Design review of the part built by this model. Coordinates are the model's own, in mm. A direction names the side the tool comes from. Give positions to 0.01 mm unless a question says otherwise; leave off trailing zeros. Order: outer loops, then holes, each group sorted by start corner. A loop starts at its lowest first (then second) coordinate and runs counter-clockwise, first axis right, second up. Notation, with made-up numbers: (49, 43.25) -> (105, 43.25) arc R23 cw to (105, 73.25) -> close; hole circle Ø8 at (72, -31). An arc over 180 degrees is marked (long way). Return JSON: item names as keys, results as strings.
```python
from build123d import *

# Parameters (mm, degrees)
SKETCH1_W           = 53.975
SKETCH1_H           = 11.1125
BOSS_EXTRUDE1_DEPTH = 38.1
FILLET1_R           = 3.175
CUT_EXTRUDE1_DEPTH  = 67.995509411
SKETCH3_R           = 2.5019
CUT_EXTRUDE2_DEPTH  = 38.1


with BuildPart() as part:
    # Sketch1 → Boss-Extrude1 (new body)
    with BuildSketch(Plane.XY):
        with Locations((26.9875, -5.55625)):
            Rectangle(SKETCH1_W, SKETCH1_H)
    extrude(amount=BOSS_EXTRUDE1_DEPTH)

    # Fillet1
    fillet1_edges = [part.edges().sort_by_distance(p)[0] for p in [
        (0, -5.55625, 38.1),
        (0, -5.55625, 0),
        (53.975, -5.55625, 0),
        (53.975, -5.55625, 38.1),
    ]]
    fillet(fillet1_edges, radius=FILLET1_R)

    # Sketch2 → Cut-Extrude1 (cut, through all)
    with BuildSketch(Plane(origin=(0, 0, 0), x_dir=(1, 0, 0), z_dir=(0, 1, 0))):
        with BuildLine():
            Line((6.35, -9.726273849), (6.35, -28.373726151))
            ThreePointArc((6.35, -28.373726151), (7.732948935, -30.63488356), (10.375852624, -30.433784883))
            Line((10.375852624, -30.433784883), (23.302722469, -21.110058732))
            ThreePointArc((23.302722469, -21.110058732), (24.356869845, -19.05), (23.302722469, -16.989941268))
            Line((23.302722469, -16.989941268), (10.375852624, -7.666215117))
            ThreePointArc((10.375852624, -7.666215117), (7.732948935, -7.46511644), (6.35, -9.726273849))
        make_face()
        with BuildLine():
            Line((18.155269838, -9.362558732), (25.501647376, -14.661259283))
            ThreePointArc((25.501647376, -14.661259283), (26.9875, -15.141200551), (28.473352624, -14.661259283))
            Line((28.473352624, -14.661259283), (35.819730162, -9.362558732))
            ThreePointArc((35.819730162, -9.362558732), (36.750915931, -6.521778917), (34.333877539, -4.7625))
            Line((34.333877539, -4.7625), (19.641122461, -4.7625))
            ThreePointArc((19.641122461, -4.7625), (17.224084069, -6.521778917), (18.155269838, -9.362558732))
        make_face()
        with BuildLine():
            Line((18.155269838, -28.737441268), (25.501647376, -23.438740717))
            ThreePointArc((25.501647376, -23.438740717), (26.9875, -22.958799449), (28.473352624, -23.438740717))
            Line((28.473352624, -23.438740717), (35.819730162, -28.737441268))
            ThreePointArc((35.819730162, -28.737441268), (36.750915931, -31.578221083), (34.333877539, -33.3375))
            Line((34.333877539, -33.3375), (19.641122461, -33.3375))
            ThreePointArc((19.641122461, -33.3375), (17.224084069, -31.578221083), (18.155269838, -28.737441268))
        make_face()
        with BuildLine():
            Line((47.625, -9.726273849), (47.625, -28.373726151))
            ThreePointArc((47.625, -28.373726151), (46.242051065, -30.63488356), (43.599147376, -30.433784883))
            Line((43.599147376, -30.433784883), (30.672277531, -21.110058732))
            ThreePointArc((30.672277531, -21.110058732), (29.618130155, -19.05), (30.672277531, -16.989941268))
            Line((30.672277531, -16.989941268), (43.599147376, -7.666215117))
            ThreePointArc((43.599147376, -7.666215117), (46.242051065, -7.46511644), (47.625, -9.726273849))
        make_face()
    extrude(amount=-CUT_EXTRUDE1_DEPTH, mode=Mode.SUBTRACT)

    # Sketch3 → Cut-Extrude2 (cut)
    with BuildSketch(Plane.XY.offset(38.1)):
        with Locations((14.2875, -5.55625)):
            Circle(SKETCH3_R)
        with Locations((39.6875, -5.55625)):
            Circle(SKETCH3_R)
    extrude(amount=-CUT_EXTRUDE2_DEPTH, mode=Mode.SUBTRACT)


solid = part.part
```
Item 1: Machinability: for faces 4 (the face through (17.24, -5.48, 31.62)), 5 (the face through (27, -5, 38.1)), which of the approach directions +Z, -Z, +X, -X, +Y, -Y give a long, thin tool a straight path to every point of the face, cutting with its end or side? Answer none if there is none.
Result set:
{"face 4": "+Y, -Y", "face 5": "+Z, +X, -X, +Y, -Y"}
Item 2: Wall thickness on L1, parallel to X at y = -3, z = 30 (3 decimals); L2, parallel to X at y = -3.5, z = 28.5 (3 decimals); L3, parallel to Z at x = 21, y = -9.5: over which ranges is each line inside the solid? List them lowest first. Write a range as [from, to].
Result set:
{"L1": "x = [0, 6.939], [10.977, 17.23], [36.745, 42.998], [47.036, 53.975]", "L2": "x = [0, 6.353], [15.713, 18.484], [35.491, 38.262], [47.622, 53.975]", "L3": "z = [0, 4.76], [11.41, 15.33], [22.77, 26.69], [33.34, 38.1]"}
Item 3: Add section A-A (z = 32). Give the boundary of the cut face in (x, y) (1 decimal), plus the area to 3 significant figures.
Result set:
{"outline": "(0, -11.1) -> (17.4, -11.1) -> (17.4, 0) -> (0, 0) -> close; (36.6, -11.1) -> (54, -11.1) -> (54, 0) -> (36.6, 0) -> close; hole circle Ø5 at (14.3, -5.6); hole circle Ø5 at (39.7, -5.6)", "area": "347 mm^2"}
Item 4: Mouldability with a two-part tool opening along Z and no side actions: class faces 1 (the face through (53.07, -5.478, 0.955)), 2 (the face through (53.07, -5.478, 37.145)), 3 (the face through (17.24, -5.48, 6.48)) as released by +Z, released by -Z, zero draft, split by the parting line, or undercut.
Result set:
{"face 1": "released by -Z", "face 2": "released by +Z", "face 3": "undercut"}
Item 5: Add section B-B (y = -9). Give the number of separate pieces and of enclosed holes in the cut face, plus the area to 3 significant figures.
Result set:
{"separate pieces": "1", "enclosed holes": "4", "area": "1,220 mm^2"}
Item 6: Add section C-C (x = 43). Give the boundary of the cut face in (y, z).
Result set:
{"outline": "(-11.11, 0) -> (0, 0) -> (0, 8.1) -> (-11.11, 8.1) -> close; (-11.11, 30) -> (0, 30) -> (0, 38.1) -> (-11.11, 38.1) -> close"}
